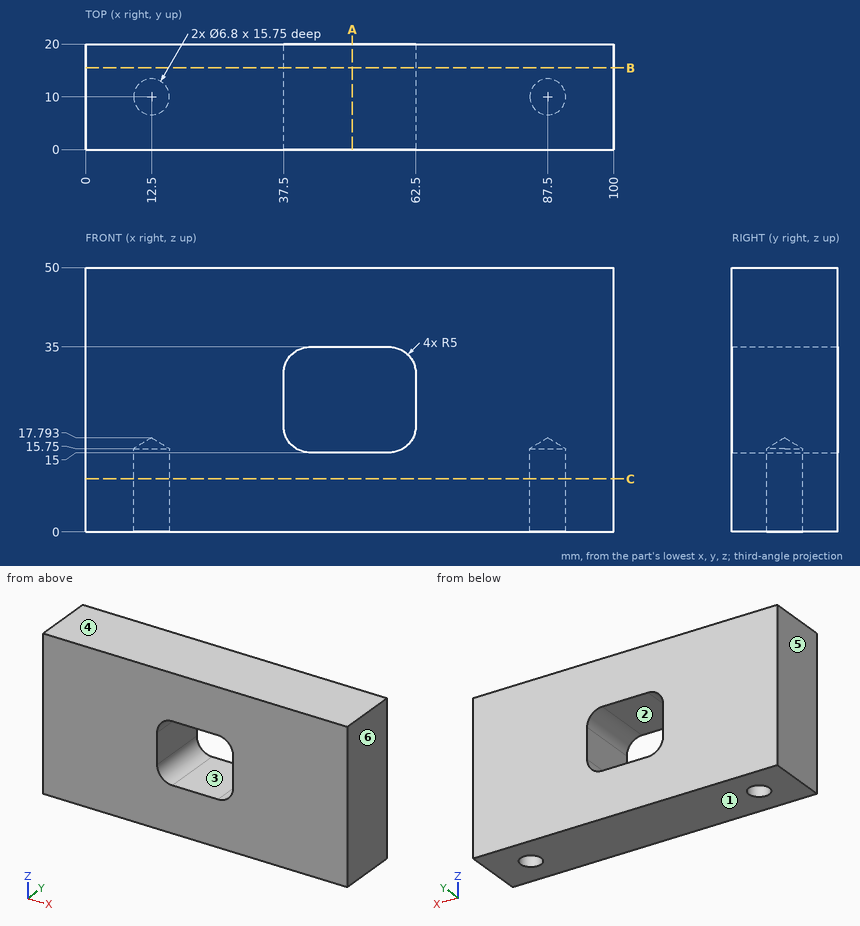
Check sheet for the drawn part. Datum: minimum x, y, z corner. Units: mm. A direction names the side the tool comes from. Round coordinates to 2 decimals unless told otherwise and drop trailing zeros. Order: outer loops, then holes, each group sorted by start corner. A loop starts at its lowest first (then second) coordinate and runs counter-clockwise, first axis right, second up. Notation, with made-up numbers: (30.25, 88.5) -> (77.25, 88.5) arc R11 cw to (77.25, 109.5) -> close; hole circle Ø8 at (21, 45.5). An arc over 180 degrees is marked (long way). Put each result on its own line as item: value. Start each with the question number.
(1) Section check B-B (y = 15.5). Enter the section's corners in (x, z), then the cut area to 3 significant figures.
(2) Section check C-C (z = 10). Enter the section's corners in (x, y).
(3) Section check A-A (x = 50.5). Enter the section's corners in (y, z), then the cut area to 3 significant figures.
(4) Depth check by flat-ended pin: pin 1 Ø5.5 at (x, y) = (87.5, 10) entering from -Z. Enter the tip coordinate at first touch or a pass-through.
(5) Draft check along X on the marked faces 3, 4, 5 and 6. Enter one of: +X half, -X half, draft (parallel to the pull), parting line (faces both ways), or undercut.
(6) Tool access check on the marked faces 1 and 2. Record the directions out of +Z, -Z, +X, -X, +Y, -Y that give a thin tool (end or side, any length) a straight path to the whole face; none if there is none.
(7) Material ranges on line 1 along X through (y, z) = (10, 6.75); line 2 along Y through (x, z) = (12.5, 10); line 3 along Z through (x, y) = (55, 4.5), recorded low to high.
Completed:
1. outline: (0, 0) -> (100, 0) -> (100, 50) -> (0, 50) -> close; hole (37.5, 20) arc R5 ccw to (42.5, 15) -> (57.5, 15) arc R5 ccw to (62.5, 20) -> (62.5, 30) arc R5 ccw to (57.5, 35) -> (42.5, 35) arc R5 ccw to (37.5, 30) -> close
1. area: 4,520 mm2
2. outline: (0, 0) -> (100, 0) -> (100, 20) -> (0, 20) -> close; hole circle Ø6.8 at (12.5, 10); hole circle Ø6.8 at (87.5, 10)
3. outline: (0, 0) -> (20, 0) -> (20, 15) -> (0, 15) -> close; (0, 35) -> (20, 35) -> (20, 50) -> (0, 50) -> close
3. area: 600 mm2
4. pin 1: stops at z = 16.14
5. face 3: undercut
5. face 4: draft
5. face 5: -X half
5. face 6: +X half
6. face 1: -Z, +X, -X, +Y, -Y
6. face 2: +Y, -Y
7. line 1: x = 0 to 9.1, 15.9 to 84.1, 90.9 to 100
7. line 2: y = 0 to 6.6, 13.4 to 20
7. line 3: z = 0 to 15, 35 to 50
